Geometry check sheet. Reference: the model listing, model coordinates, mm. A direction names the side the tool comes from. Coordinates: 2 decimals unless noted, no trailing zeros. Order: outer loops, then holes, each group sorted by start corner. A loop starts at its lowest first (then second) coordinate and runs counter-clockwise, first axis right, second up. Notation, with made-up numbers: (-33, -16.75) - (-21, -16.75) arc R16 cw to (-21, -12.75) - close; hole circle Ø9 at (56.5, -17). An arc over 180 degrees is marked (long way). Put each result on its own line as item: value.
from build123d import *

# Parameters (mm, degrees)
SKETCH1_W               = 63.5
SKETCH1_H               = 38.1
SKETCH1_R               = 2.6543
BOSS_EXTRUDE1_DEPTH     = 9.525
CUT_EXTRUDE2_DEPTH      = 39.232062788
CUT_EXTRUDE2_DEPTH_BACK = 4.7625
SKETCH4_R               = 5
CUT_EXTRUDE3_DEPTH      = 39.232062788
CUT_EXTRUDE3_DEPTH_BACK = 39.232062788
SKETCH5_R               = 2.1


with BuildPart() as part:
    # Sketch1 → Boss-Extrude1 (new body)
    with BuildSketch(Plane.XY):
        Rectangle(SKETCH1_W, SKETCH1_H)
        with Locations(Location((-19.875, 11.875, 0), (0, 0, 180))):
            Circle(SKETCH1_R, mode=Mode.SUBTRACT)
        with Locations(Location((-19.875, -11.875, 0), (0, 0, 180))):
            Circle(SKETCH1_R, mode=Mode.SUBTRACT)
        with Locations(Location((19.875, -11.875, 0), (0, 0, 180))):
            Circle(SKETCH1_R, mode=Mode.SUBTRACT)
        with Locations(Location((19.875, 11.875, 0), (0, 0, 180))):
            Circle(SKETCH1_R, mode=Mode.SUBTRACT)
    extrude(amount=BOSS_EXTRUDE1_DEPTH)

    # Sketch4 → Cut-Extrude2 (cut, two sides: drawn at the far end of the back side and taken through both)
    with BuildSketch(Plane.XY.offset(9.525).offset(-CUT_EXTRUDE2_DEPTH_BACK)):
        with Locations(Location((19.875, -11.875, 0), (0, 0, 180))):
            Circle(SKETCH4_R)
        with Locations(Location((19.875, 11.875, 0), (0, 0, 180))):
            Circle(SKETCH4_R)
        with Locations(Location((-19.875, 11.875, 0), (0, 0, 180))):
            Circle(SKETCH4_R)
        with Locations(Location((-19.875, -11.875, 0), (0, 0, 180))):
            Circle(SKETCH4_R)
    extrude(amount=CUT_EXTRUDE2_DEPTH + CUT_EXTRUDE2_DEPTH_BACK, mode=Mode.SUBTRACT)

    # Sketch5 → Cut-Extrude3 (cut, two sides: drawn at the far end of the back side and taken through both)
    with BuildSketch(Plane(origin=(0, 0, 0), x_dir=(1, 0, 0), z_dir=(0, 1, 0)).offset(-CUT_EXTRUDE3_DEPTH_BACK)):
        with Locations(Location((-11.1125, -4.7625, 0), (0, 0, 270))):
            Circle(SKETCH5_R)
        with Locations(Location((11.1125, -4.7625, 0), (0, 0, 90))):
            Circle(SKETCH5_R)
    extrude(amount=CUT_EXTRUDE3_DEPTH + CUT_EXTRUDE3_DEPTH_BACK, mode=Mode.SUBTRACT)


solid = part.part
Q1. Thickness scan on L1, parallel to X at y = 3, z = 6; L2, parallel to X at y = 13.5, z = 5.5; L3, parallel to Y at x = 18.5, z = 7.5. Record the ranges inside material, lowest first. Write a range as [from, to].
Answer block:
L1: x = [-31.75, -12.81], [-9.42, 9.42], [12.81, 31.75]
L2: x = [-31.75, -24.6], [-15.15, -13.08], [-9.15, 9.15], [13.08, 15.15], [24.6, 31.75]
L3: y = [-19.05, -16.68], [-7.07, 7.07], [16.68, 19.05]
Q2. Access from +Z, -Z, +X, -X, +Y, -Y to the whole of each face (thin tool, end or side, straight path). Record for faces 1 (the flat face through (17.7, -9.7, 4.762)), 2 (the cylindrical face through (9.342, -0.267, 3.634)).
Answer block:
face 1: +Z
face 2: +Y, -Y
Q3. Section check A-A on z = 5.5. Record the boundary of the cut face in (x, y) (3 decimals), then the cut area to 3 significant figures.
Answer block:
outline: (-31.75, -19.05) - (-13.079, -19.05) - (-13.079, 19.05) - (-31.75, 19.05) - close; (-9.146, -19.05) - (9.146, -19.05) - (9.146, 19.05) - (-9.146, 19.05) - close; (13.079, -19.05) - (31.75, -19.05) - (31.75, 19.05) - (13.079, 19.05) - close; hole circle Ø10 at (-19.875, -11.875); hole circle Ø10 at (-19.875, 11.875); hole circle Ø10 at (19.875, -11.875); hole circle Ø10 at (19.875, 11.875)
area: 1,810 mm^2
Q4. Draft check along X on faces 3 (the flat face through (0, 0, 0)), 4 (the cylindrical face through (17.423, -10.858, 2.348)), 5 (the flat face through (31.75, 0, 5)), 6 (the flat face through (-31.75, 0, 5)). Enter one of: pulls with the +X half, pulls with the -X half, needs draft (parallel to the pull), parting line crosses it, or undercut.
Answer block:
face 3: needs draft
face 4: undercut
face 5: pulls with the +X half
face 6: pulls with the -X half
Q5. Depth check by flat-ended pin: pin 1 Ø4 at (x, z) = (-11.11, 4.76) entering from -Y; pin 2 Ø5 at (x, y) = (20.5, 10.5) entering from +Z. Enter the tip coordinate at first touch or a pass-through.
Answer block:
pin 1: passes through
pin 2: stops at z = 4.76
Q6. Section check B-B on x = -20. State how many separate pieces and enclosed holes the cut face has, then the cut area to 3 significant figures.
Answer block:
separate pieces: 3
enclosed holes: 0
area: 217 mm^2
